Geometry check sheet. Reference: the model listing, model coordinates, mm. A direction names the side the tool comes from. Round coordinates to 2 decimals unless told otherwise and drop trailing zeros. Order: outer loops, then holes, each group sorted by start corner. A loop starts at its lowest first (then second) coordinate and runs counter-clockwise, first axis right, second up. Notation, with made-up numbers: (9, 35) -> (35, 35) arc R19 ccw to (35, 65) -> close; hole circle Ø11 at (-31, 7.25). An arc over 180 degrees is marked (long way). Answer as a JSON object with one key per item and string values. Group by question number.
from build123d import *

# Parameters (mm, degrees)
SKETCH001_R         = 14.291544
POCKET_DEPTH        = 31.151
REVOLUTION001_ANGLE = 30
REVOLUTION002_ANGLE = 30
REVOLUTION003_ANGLE = 30
REVOLUTION004_ANGLE = 30
SKETCH006_W         = 0.8
SKETCH006_H         = 2.14163
POCKET001_DEPTH     = 107.126588
POLARPATTERN_COUNT  = 4


with BuildPart() as part:
    # Sketch → Revolution (revolve)
    with BuildSketch(Plane.XZ):
        with BuildLine():
            Line((-5.3, 0), (-5.3, 6))
            ThreePointArc((-5.3, 6), (-4.244457, 6.413224), (-3.75, 7.433241))
            Line((-3.775, 18.6), (-3.75, 7.433241))
            Line((-3.775, 20.95), (-3.775, 18.6))
            Line((-3.075, 20.95), (-3.775, 20.95))
            Line((-3.075, 21.55), (-3.075, 20.95))
            Line((-2.7, 21.55), (-3.075, 21.55))
            Line((-2.7, 21.55), (-2.55, 28.55))
            Line((-2.55, 28.55), (-1.45, 31.15))
            Line((-1.45, 31.15), (-3.764164, 31.15))
            Line((-3.764164, 31.15), (-6.55502, 23.635956))
            Line((-6.55502, 23.635956), (-6.55502, 10.794422))
            Line((-6.55502, 10.794422), (-8, 7.60349))
            Line((-8, 7.60349), (-8, 0))
            Line((-5.3, 0), (-8, 0))
        make_face()
    revolve(axis=Axis((0, 0, 0), (0, 0, 1)))

    # Sketch001 (on Face8 of Revolution) → Pocket (cut, through all)
    with BuildSketch(Plane(origin=(0, 0, 0), x_dir=(1, 0, 0), z_dir=(0, 0, -1))):
        Circle(SKETCH001_R)
        Polygon((8.5, 0), (4.25, 7.361216), (-4.25, 7.361216), (-8.5, 0), (-4.25, -7.361216), (4.25, -7.361216), align=None, mode=Mode.SUBTRACT)
    extrude(amount=-POCKET_DEPTH, mode=Mode.SUBTRACT)

    # Sketch002 → Revolution001 (revolve, symmetric)
    with BuildSketch(Plane.XZ) as revolution001_sk:
        Polygon((-5.5, 0), (-4.5, 0.6), (-5.5, 1.2), (-6.5, 1.2), (-6.5, 0), align=None)
        Polygon((-5.5, 1.5), (-4.5, 2.1), (-5.5, 2.7), (-6.5, 2.7), (-6.5, 1.5), align=None)
        Polygon((-5.5, 3), (-4.5, 3.6), (-5.5, 4.2), (-6.5, 4.2), (-6.5, 3), align=None)
    revolve(axis=Axis((0, 0, 0), (0, 0, 1)), revolution_arc=REVOLUTION001_ANGLE / 2)
    revolve(revolution001_sk.sketch, axis=Axis((0, 0, 0), (0, 0, -1)), revolution_arc=REVOLUTION001_ANGLE / 2)

    # Sketch003 → Revolution002 (revolve, symmetric)
    with BuildSketch(Plane(origin=(0, 0, 0.375), x_dir=(0, 1, 0), z_dir=(1, 0, 0))) as revolution002_sk:
        Polygon((-5.5, 0), (-4.5, 0.6), (-5.5, 1.2), (-6.5, 1.2), (-6.5, 0), align=None)
        Polygon((-5.5, 1.5), (-4.5, 2.1), (-5.5, 2.7), (-6.5, 2.7), (-6.5, 1.5), align=None)
        Polygon((-5.5, 3), (-4.5, 3.6), (-5.5, 4.2), (-6.5, 4.2), (-6.5, 3), align=None)
    revolve(axis=Axis((0, 0, 0.375), (0, 0, 1)), revolution_arc=REVOLUTION002_ANGLE / 2)
    revolve(revolution002_sk.sketch, axis=Axis((0, 0, 0.375), (0, 0, -1)), revolution_arc=REVOLUTION002_ANGLE / 2)

    # Sketch004 → Revolution003 (revolve, symmetric)
    with BuildSketch(Plane(origin=(0, 0, 0.75), x_dir=(-1, 0, 0), z_dir=(0, 1, 0))) as revolution003_sk:
        Polygon((-5.5, 0), (-4.5, 0.6), (-5.5, 1.2), (-6.5, 1.2), (-6.5, 0), align=None)
        Polygon((-5.5, 1.5), (-4.5, 2.1), (-5.5, 2.7), (-6.5, 2.7), (-6.5, 1.5), align=None)
        Polygon((-5.5, 3), (-4.5, 3.6), (-5.5, 4.2), (-6.5, 4.2), (-6.5, 3), align=None)
    revolve(axis=Axis((0, 0, 0.75), (0, 0, 1)), revolution_arc=REVOLUTION003_ANGLE / 2)
    revolve(revolution003_sk.sketch, axis=Axis((0, 0, 0.75), (0, 0, -1)), revolution_arc=REVOLUTION003_ANGLE / 2)

    # Sketch005 → Revolution004 (revolve, symmetric)
    with BuildSketch(Plane(origin=(0, 0, 1.125), x_dir=(0, -1, 0), z_dir=(-1, 0, 0))) as revolution004_sk:
        Polygon((-5.5, 0), (-4.5, 0.6), (-5.5, 1.2), (-6.5, 1.2), (-6.5, 0), align=None)
        Polygon((-5.5, 1.5), (-4.5, 2.1), (-5.5, 2.7), (-6.5, 2.7), (-6.5, 1.5), align=None)
        Polygon((-5.5, 3), (-4.5, 3.6), (-5.5, 4.2), (-6.5, 4.2), (-6.5, 3), align=None)
    revolve(axis=Axis((0, 0, 1.125), (0, 0, 1)), revolution_arc=REVOLUTION004_ANGLE / 2)
    revolve(revolution004_sk.sketch, axis=Axis((0, 0, 1.125), (0, 0, -1)), revolution_arc=REVOLUTION004_ANGLE / 2)

    # Sketch006 (on Face5 of Revolution004) → Pocket001 (cut, through all)
    with BuildSketch(Plane(origin=(0, 0, 31.15), x_dir=(-1, 0, 0), z_dir=(0, 0, 1))):
        with Locations((0, 1.929185)):
            Rectangle(SKETCH006_W, SKETCH006_H)
    pocket001 = extrude(amount=-POCKET001_DEPTH, mode=Mode.SUBTRACT)

    # PolarPattern: Pocket001 ×4 about axis
    polarpattern_axis = Axis((0, 0, 31.15), (0, 0, 1))
    for i in range(1, POLARPATTERN_COUNT):
        add(pocket001.rotate(polarpattern_axis, i * 360 / POLARPATTERN_COUNT), mode=Mode.SUBTRACT)


solid = part.part
Item 1: Thickness scan on L1, parallel to X at y = 0, z = 21.25 (3 decimals); L2, parallel to Y at x = 0, z = 19.3 (3 decimals). Record the ranges inside material, lowest first.
Item 2: Mould release check, pull along Y, two halves, no side actions. Record for faces 1 (the flat face through (6.35, 3.72, 4.44)), 2 (the cylindrical face through (-8, 0, 4)), 3 (the conical face through (-4.906, 0.018, 2.343)): pulls with the +Y half, pulls with the -Y half, needs draft (parallel to the pull), parting line crosses it, or undercut.
Item 3: Depth check by flat-ended pin: pin 1 Ø1.5 at (x, y) = (1, -2) entering from -Z; pin 2 Ø4 at (x, z) = (5, 10) entering from -Y; pin 3 Ø1.8 at (y, z) = (2.5, 25) entering from -X. Enter the tip coordinate at first touch or a pass-through.
Item 4: Sectioned sample at A-A, the plane z = 22.5. Enter the section's corners in (x, y), then the cut area to 3 significant figures.
Item 5: Set-up check for faces 4 (the flat face through (2.7, -0.4, 27.8)), 5 (the cylindrical face through (0.67, 3, 21.25)), 6 (the conical face through (4.906, 0.018, 1.593)): record each of +Z, -Z, +X, -X, +Y, -Y from which the full face is reachable in a straight line by a thin tool's end or side.
Item 6: Sectioned sample at B-B, the plane z = 29. Enter the section's corners in (x, y), then the cut area to 3 significant figures.
Result:
{
 "1": {"L1": "x = -6.555 to -3.075, 3.075 to 6.555", "L2": "y = -6.555 to -3.775, 3.775 to 6.555"},
 "2": {"face 1": "pulls with the +Y half", "face 2": "parting line crosses it", "face 3": "undercut"},
 "3": {"pin 1": "stops at z = 21.55", "pin 2": "stops at y = -6.65", "pin 3": "stops at x = -6"},
 "4": {"outline": "circle Ø13.11 at (0, 0); hole (-3, -0.4) -> (-2.65, -0.4) arc R2.68 ccw to (-0.4, -2.65) -> (-0.4, -3) -> (0.4, -3) -> (0.4, -2.65) arc R2.68 ccw to (2.65, -0.4) -> (3, -0.4) -> (3, 0.4) -> (2.65, 0.4) arc R2.68 ccw to (0.4, 2.65) -> (0.4, 3) -> (-0.4, 3) -> (-0.4, 2.65) arc R2.68 ccw to (-2.65, 0.4) -> (-3, 0.4) -> close", "area": "111 mm2"},
 "5": {"face 4": "+Z, -Z", "face 5": "-Z", "face 6": "none"},
 "6": {"outline": "circle Ø9.13 at (0, 0); hole (-3, -0.4) -> (-2.33, -0.4) arc R2.36 ccw to (-0.4, -2.33) -> (-0.4, -3) -> (0.4, -3) -> (0.4, -2.33) arc R2.36 ccw to (2.33, -0.4) -> (3, -0.4) -> (3, 0.4) -> (2.33, 0.4) arc R2.36 ccw to (0.4, 2.33) -> (0.4, 3) -> (-0.4, 3) -> (-0.4, 2.33) arc R2.36 ccw to (-2.33, 0.4) -> (-3, 0.4) -> close", "area": "45.8 mm2"}
}
